Autodesk Inventor part; units mm, degrees
ref_plane "YZ Plane" through (0, 0, 0) normal (1, 0, 0) x (0, 1, 0)
ref_plane "XZ Plane" through (0, 0, 0) normal (0, 1, 0) x (-1, 0, 0)
ref_plane "XY Plane" through (0, 0, 0) normal (0, 0, 1) x (1, 0, 0)
sketch "Sketch1" plane through (0, 0, 0) normal (0, 0, 1) x (1, 0, 0)
  circle A0 centre (0, 0) radius 16
  dimension "d0" = 32
extrude "Extrusion1" add sketch "Sketch1" along normal blind 21
sketch "Sketch2" plane through (0, 0, 21) normal (0, 0, 1) x (1, 0, 0)
  circle A0 centre (0, 0) radius 14.5
  dimension "d3" = 29
extrude "Extrusion2" add sketch "Sketch2" along normal blind 1.5
sketch "Sketch3" plane through (0, 0, 22.5) normal (0, 0, 1) x (1, 0, 0)
  circle A0 centre (0, 0) radius 16
  dimension "d6" = 32
extrude "Extrusion3" add sketch "Sketch3" along normal blind 3
sketch "Sketch4" plane through (0, 0, 25.5) normal (0, 0, 1) x (1, 0, 0)
  circle A0 centre (0, 0) radius 14.5
  dimension "d9" = 29
extrude "Extrusion4" add sketch "Sketch4" along normal blind 1.5
sketch "Sketch5" plane through (0, 0, 27) normal (0, 0, 1) x (1, 0, 0)
  circle A0 centre (0, 0) radius 16
  dimension "d12" = 32
extrude "Extrusion5" add sketch "Sketch5" along normal blind 3
sketch "Sketch6" plane through (0, 0, 30) normal (0, 0, 1) x (1, 0, 0)
  circle A0 centre (0, 0) radius 16
  dimension "d15" = 32
extrude "Extrusion6" add sketch "Sketch6" along normal blind 2 draft -80
sketch "Sketch7" plane through (0, 0, 0) normal (0, 0, -1) x (-1, 0, 0)
  circle A0 centre (0, 0) radius 13
  dimension "d18" = 26
extrude "Extrusion7" cut sketch "Sketch7" against normal blind 10
sketch "Sketch8" plane through (0, 0, 10) normal (0, 0, -1) x (-1, 0, 0)
  circle A0 centre (0, 0) radius 10
  dimension "d21" = 20
extrude "Extrusion8" cut sketch "Sketch8" against normal blind 14
sketch "Sketch9" plane through (0, 0, 0) normal (0, 1, 0) x (-1, 0, 0)
  circle A0 centre (0, 16) radius 2.5
  point P0 (0, 0)
  dimension "d24" = 5
extrude "Extrusion9" cut sketch "Sketch9" along normal mid plane 32
properties part number "piston"
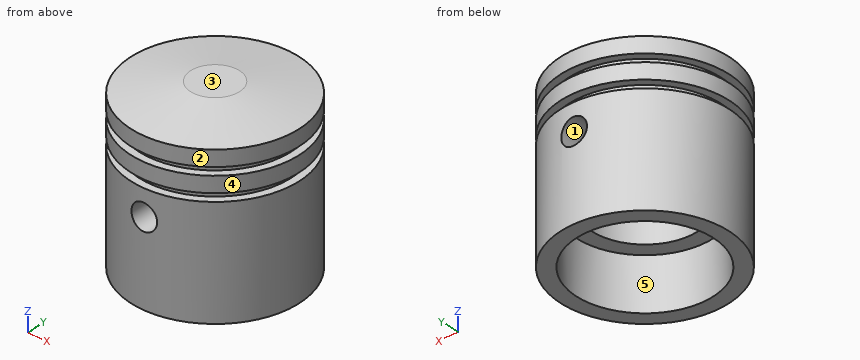
Geometry: final body of the model. Coordinates: model frame, mm. Face numbers are marked on the shaded views. A direction names the side the tool comes from. Give positions to 0.01 mm unless a question says otherwise; leave off trailing zeros. Write each loop counter-clockwise with the first axis right and the second up, starting at its lowest first coordinate (ties: lowest second). Pieces come first, ordered by that corner, then holes. Notation, with made-up numbers: (-12, 66.25) - (26, 66.25) arc R28 ccw to (26, 98.25) - close; hole circle Ø3 at (-12, 36.25). An arc over 180 degrees is marked (long way). Return JSON: item names as keys, results as strings. Group by question number.
1) Section D-D on x = 0. State how many separate pieces and enclosed holes the cut face has, plus the area to 3 significant figures.
2) First-contact query: P1, Ø3, axis at x = 0, z = 16, coming from the +Y side; P2, Ø8, axis at x = -2.5, y = 2.5, coming from the -Z side; P3, Ø1, axis at x = -6.5, y = -8.5, coming from the +Z side; P4, Ø3, axis at x = -5, z = 17.5, coming from the +Y side. Flat tips, straight axial feed; report the tip coordinate or a pass-through.
3) Line query: line 1 (Y direction, x = 6.5, z = 20); line 2 (X direction, y = -0.5, z = 18.5); line 3 (Y direction, x = 7, z = 4.5). Output: solid intervals per line, ascending.
4) Mould query, pull axis Z, two halves, no side actions, for the marked faces 1, 2 and 3. Classes: released by +Z, released by -Z, zero draft, split by the parting line, or undercut.
5) Section B-B on z = 12.5. Return the cut outline in (x, y).
6) Set-up query: the marked faces 4 and 5. Return all of +Z, -Z, +X, -X, +Y, -Y with unobstructed straight access to the full face (end or side cutting, diameter ignored); none if empty.
7) Section C-C on z = 16. Return the cut outline in (x, y), plus the area to 3 significant figures.
Filled in:
{
 "1": {"separate pieces": "3", "enclosed holes": "0", "area": "392 mm^2"},
 "2": {"P1": "passes through", "P2": "stops at z = 24", "P3": "stops at z = 31.02", "P4": "stops at y = 15.61"},
 "3": {"line 1": "y = -14.62 to -7.6, 7.6 to 14.62", "line 2": "x = -15.99 to -9.99, 9.99 to 15.99", "line 3": "y = -14.39 to -10.95, 10.95 to 14.39"},
 "4": {"face 1": "undercut", "face 2": "zero draft", "face 3": "released by +Z"},
 "5": {"outline": "circle Ø32 at (0, 0); hole circle Ø20 at (0, 0)"},
 "6": {"face 4": "+Z, -Z", "face 5": "-Z"},
 "7": {"outline": "(-2.5, -15.8) - (-2.5, -9.68) arc R10 cw to (-2.5, 9.68) - (-2.5, 15.8) arc R16 ccw to start; (2.5, -15.8) arc R16 ccw to (2.5, 15.8) - (2.5, 9.68) arc R10 cw to (2.5, -9.68) - close", "area": "430 mm^2"}
}
